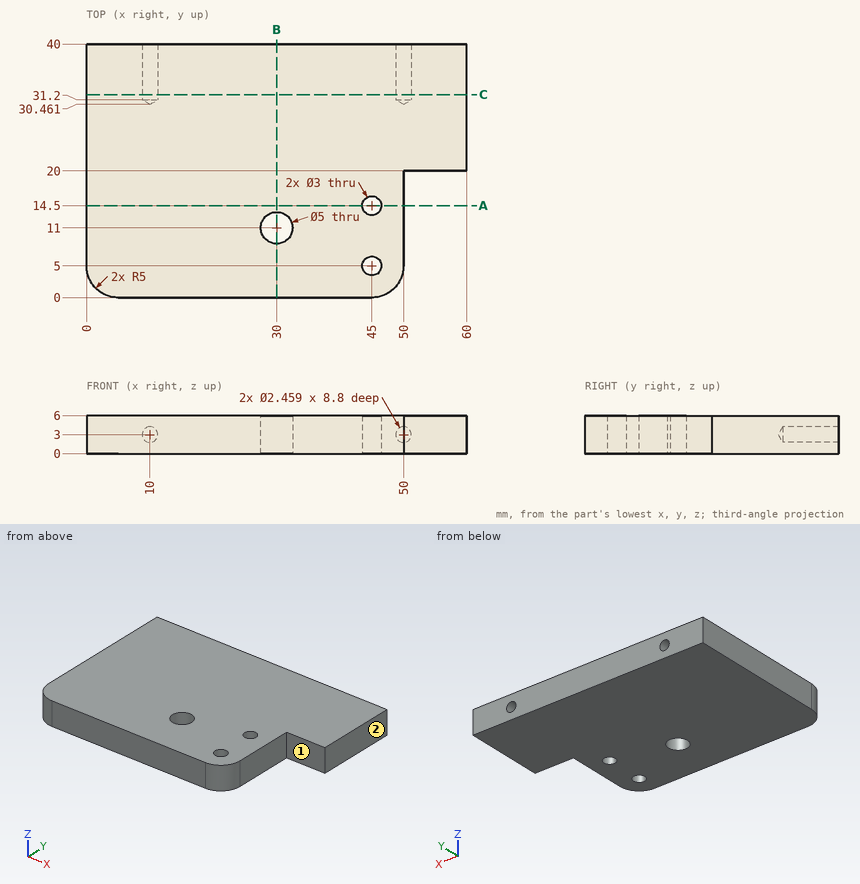
Job drawing, mm, ordinate dimensions from the low corner. One solid piece. A direction names the side the tool comes from. Give positions to 0.01 mm unless a question says otherwise; leave off trailing zeros. Loops run counter-clockwise (first coordinate to the right, second up) from the corner with the lowest first, then second, coordinate; pieces in that order, holes last. Notation, with made-up numbers: M -13,49 L 23,49 A14 cw 23,67 Z; hole C 20,66 d10. An arc over 180 degrees is marked long. Return JSON: item names as keys, results as strings.
1) Saw through at C-C, the plane y = 32. List the corners of the cut face in (x, z).
Calculated:
{"outline": "M 0,0 L 60,0 L 60,6 L 0,6 Z; hole C 10,3 d2.46; hole C 50,3 d2.46"}
2) 3-axis set-ups, long thin cutter, end or side, ignore diameter. For the marked faces 1 and 2: which of +Z, -Z, +X, -X, +Y, -Y reach the whole face in a straight line?
Calculated:
{"face 1": "+Z, -Z, +X, -Y", "face 2": "+Z, -Z, +X, +Y, -Y"}
3) Drill centre lines: line 1 (Y direction, x = 45, z = 1.4); line 2 (X direction, y = 35.5, z = 3); line 3 (X direction, y = 14.5, z = 2.5). Where is each one in solid material? Low to high.
Calculated:
{"line 1": "y = 0 to 3.5, 6.5 to 13, 16 to 40", "line 2": "x = 0 to 8.77, 11.23 to 48.77, 51.23 to 60", "line 3": "x = 0 to 43.5, 46.5 to 50"}
4) Flat gauge pins, fed straight in: pin 1 Ø3 at (x, z) = (54, 2.5) entering from -Y; pin 2 Ø1.8 at (y, z) = (10, 2.5) entering from +X; pin 3 Ø4.5 at (x, y) = (30, 11) entering from -Z (3 decimals). Where does each tip first touch, or does it go through?
Calculated:
{"pin 1": "stops at y = 20", "pin 2": "stops at x = 50", "pin 3": "passes through"}
5) Saw through at A-A, the plane y = 14.5. List the corners of the cut face in (x, z).
Calculated:
{"outline": "M 0,0 L 43.5,0 L 43.5,6 L 0,6 Z; M 46.5,0 L 50,0 L 50,6 L 46.5,6 Z"}
6) Saw through at B-B, the plane x = 30. List the corners of the cut face in (y, z).
Calculated:
{"outline": "M 0,0 L 8.5,0 L 8.5,6 L 0,6 Z; M 13.5,0 L 40,0 L 40,6 L 13.5,6 Z"}
